Input: part model. Units: mm. Frame: model coordinates. Face numbers are marked on the shaded views. Coordinates: 2 decimals unless noted, no trailing zeros. Loops run counter-clockwise (first coordinate to the right, second up) from the corner with the lowest first, then second, coordinate; pieces in that order, holes last. Notation, with made-up numbers: (35, 72) - (73, 72) arc R18 ccw to (73, 81) - close; hole circle Ø8 at (-25, 23). An arc over 180 degrees is marked (long way). Write item = value, one per line. Start each with the question number.
from build123d import *

# Parameters (mm, degrees)
F1_DEPTH = 6.3
F2_R     = 0.4
F5_D     = 9


with BuildPart() as f1:
    # F0 (on Top) → F1 (new body)
    with BuildSketch(Plane.XY):
        Polygon((7.3900834456, 0), (3.6950417228, 6.4), (-3.6950417228, 6.4), (-7.3900834456, 0), (-3.6950417228, -6.4), (3.6950417228, -6.4), align=None)
    extrude(amount=F1_DEPTH)

    # F2
    f2_edges = [f1.edges().sort_by_distance(p)[0] for p in [
        (-3.695042, -6.4, 3.15),
        (3.695042, -6.4, 3.15),
        (7.390083, 0, 3.15),
        (3.695042, 6.4, 3.15),
        (-3.695042, 6.4, 3.15),
        (-7.390083, 0, 3.15),
    ]]
    fillet(f2_edges, radius=F2_R)

    # F3 (on Right) → F4 (revolve, cut)
    with BuildSketch(Plane.YZ):
        Polygon((9.5, 6.3), (6.5, 6.3), (9.5, 3.3), align=None)
        Polygon((9.5, 3), (6.5, 0), (9.5, 0), align=None)
    revolve(axis=Axis((0, 0, 10.4480586015), (0, 0, -1)), mode=Mode.SUBTRACT)

    # F5 (through all)
    with Locations(Plane(origin=(0, 0, 0), x_dir=(1, 0, 0), z_dir=(0, 0, -1))):
        with Locations((0, 0)):
            Hole(F5_D / 2)


solid = f1.part
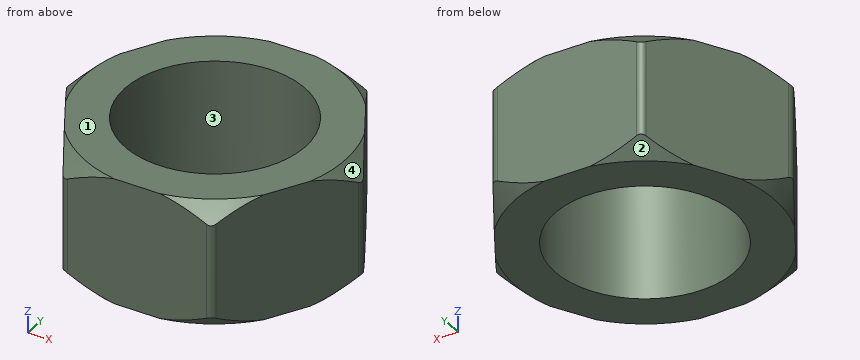
Item 1: Cut plane A-A on x = 0. Return loops of the section in (y, z), plus the area to 3 significant figures.
Item 2: Pin query (flat end, axial travel): pin 1 (2 mm diameter, centred on y = 0.5, z = 5, fed in from -X); pin 2 (3 mm diameter, centred on y = -4, z = 5.5, fed in from +X). Return the tip coordinate at first contact, or that it passes through.
Item 3: Ray query, line 1 (Y direction, x = 0, z = 4); line 2 (X direction, y = -1, z = 5.75); line 3 (X direction, y = 2.5, z = 1.75). Return the intervals inside material, ascending.
Item 4: Cut plane B-B on y = 0. Return loops of the section in (x, z).
Item 5: Cut plane C-C on z = 2.25. Return loops of the section in (x, y), plus the area to 3 significant figures.
Item 6: Pull-direction query (X, two-part tool) for the marked faces 1, 2, 3 and 4; classes: pulls with the +X half, pulls with the -X half, needs draft (parallel to the pull), parting line crosses it, or undercut.
Recorded:
q1.outline = (-6.4, 0) - (-4.5, 0) - (-4.5, 6.3) - (-6.4, 6.3) - close; (4.5, 0) - (6.4, 0) - (6.4, 6.3) - (4.5, 6.3) - close
q1.area = 23.9 mm²
q2.pin_1 = -7.33
q2.pin_2 = 5.95
q3.line_1 = -6.4 to -4.5, 4.5 to 6.4
q3.line_2 = -6.81 to -4.39, 4.39 to 6.81
q3.line_3 = -5.95 to -3.74, 3.74 to 5.95
q4.outline = (-7.33, 0.83) - (-6.5, 0) - (-4.5, 0) - (-4.5, 6.3) - (-6.5, 6.3) - (-7.33, 5.47) - close; (4.5, 0) - (6.5, 0) - (7.33, 0.83) - (7.33, 5.47) - (6.5, 6.3) - (4.5, 6.3) - close
q5.outline = (-7.27, -0.2) - (-3.81, -6.2) arc R0.4 ccw to (-3.46, -6.4) - (3.46, -6.4) arc R0.4 ccw to (3.81, -6.2) - (7.27, -0.2) arc R0.4 ccw to (7.27, 0.2) - (3.81, 6.2) arc R0.4 ccw to (3.46, 6.4) - (-3.46, 6.4) arc R0.4 ccw to (-3.81, 6.2) - (-7.27, 0.2) arc R0.4 ccw to start; hole circle Ø9 at (0, 0)
q5.area = 78.2 mm²
q6.face_1 = needs draft
q6.face_2 = pulls with the -X half
q6.face_3 = undercut
q6.face_4 = pulls with the +X half
